from build123d import *

# Parameters (mm, degrees)
F1_DEPTH = 3.175


# Not quite as in the source:
# - a length typed as a fraction of an inch, garbled in the dataset ("3 / 203.2 mm" for 3/8 in), is restored


with BuildPart() as f1:
    # F0 (on Top) → F1 (new body)
    with BuildSketch(Plane.XY):
        with BuildLine():
            ThreePointArc((-41.4974734498, 12.7), (-32.5172173287, 8.9802561211), (-28.7974734498, 0))
            Line((-28.7974734498, 0), (32.2387265502, 0))
            ThreePointArc((32.2387265502, 0), (35.9584704291, 8.9802561211), (44.9387265502, 12.7))
            Line((44.9387265502, 12.7), (-41.4974734498, 12.7))
        make_face()
        with BuildLine():
            ThreePointArc((-41.4974734498, -4.7625), (-44.8650694952, 3.3675960454), (-36.7349734498, 0))
            Line((-36.7349734498, 0), (-28.7974734498, 0))
            ThreePointArc((-28.7974734498, 0), (-32.5172173287, 8.9802561211), (-41.4974734498, 12.7))
            ThreePointArc((-41.4974734498, 12.7), (-54.1974734498, 0), (-41.4974734498, -12.7))
            Line((-41.4974734498, -12.7), (-41.4974734498, -4.7625))
        make_face()
        with BuildLine():
            Line((-28.7974734498, 0), (-36.7349734498, 0))
            ThreePointArc((-36.7349734498, 0), (-38.1298774044, -3.3675960454), (-41.4974734498, -4.7625))
            Line((-41.4974734498, -4.7625), (-41.4974734498, -12.7))
            ThreePointArc((-41.4974734498, -12.7), (-32.5172173287, -8.9802561211), (-28.7974734498, 0))
        make_face()
        with BuildLine():
            Line((32.2387265502, 0), (-28.7974734498, 0))
            ThreePointArc((-28.7974734498, 0), (-32.5172173287, -8.9802561211), (-41.4974734498, -12.7))
            Line((-41.4974734498, -12.7), (44.9387265502, -12.7))
            ThreePointArc((44.9387265502, -12.7), (35.9584704291, -8.9802561211), (32.2387265502, 0))
        make_face()
        with BuildLine():
            ThreePointArc((44.9387265502, 12.7), (35.9584704291, 8.9802561211), (32.2387265502, 0))
            ThreePointArc((32.2387265502, 0), (35.9584704291, -8.9802561211), (44.9387265502, -12.7))
            ThreePointArc((44.9387265502, -12.7), (53.9189826713, -8.9802561211), (57.6387265502, 0))
            ThreePointArc((57.6387265502, 0), (53.9189826713, 8.9802561211), (44.9387265502, 12.7))
        make_face()
        with BuildLine():
            ThreePointArc((49.7012265502, 0), (44.9387265502, -4.7625), (40.1762265502, 0))
            ThreePointArc((40.1762265502, 0), (44.9387265502, 4.7625), (49.7012265502, 0))
        make_face(mode=Mode.SUBTRACT)
    extrude(amount=F1_DEPTH)


solid = f1.part
Geometry check sheet. Reference: the model listing, model coordinates, mm. Give positions to 0.01 mm unless a question says otherwise; leave off trailing zeros. Write each loop counter-clockwise with the first axis right and the second up, starting at its lowest first coordinate (ties: lowest second). Pieces come first, ordered by that corner, then holes. Notation, with made-up numbers: (22.25, 10.25) - (80.25, 10.25) arc R28 cw to (80.25, 32.25) - close; hole circle Ø2 at (81, 89). An arc over 180 degrees is marked (long way). Put each result on its own line as item: value.
1. Draft check along X on faces 1 (the flat face through (1, 0, 0)), 2 (the cylindrical face through (-54.194, 0.279, 1.565)), 3 (the cylindrical face through (-46.255, -0.209, 1.565)). Enter one of: +X half, -X half, draft (parallel to the pull), parting line (faces both ways), or undercut.
Ans:
face 1: draft
face 2: -X half
face 3: undercut
2. Thickness scan on line 1 (X direction, y = 3.75, z = 1.35); line 2 (X direction, y = -0.5, z = 2.5); line 3 (Y direction, x = 48.5, z = 2.05). Record the ranges inside material, lowest first.
Ans:
line 1: x = -53.63 to -44.43, -38.56 to 42, 47.87 to 57.07
line 2: x = -54.19 to -46.23, -36.76 to 40.2, 49.67 to 57.63
line 3: y = -12.19 to -3.16, 3.16 to 12.19
3. Sectioned sample at A-A, the plane z = 1.5. Enter the section's corners in (x, y) (1 decimal).
Ans:
outline: (-41.5, -12.7) - (44.9, -12.7) arc R12.7 ccw to (44.9, 12.7) - (-41.5, 12.7) arc R12.7 ccw to start; hole circle Ø9.5 at (-41.5, 0); hole circle Ø9.5 at (44.9, 0)
4. Sectioned sample at B-B, the plane y = -3.25. Enter the section's corners in (x, z) (1 decimal), plus the area to 3 significant figures.
Ans:
outline: (-53.8, 0) - (-45, 0) - (-45, 3.2) - (-53.8, 3.2) - close; (-38, 0) - (41.5, 0) - (41.5, 3.2) - (-38, 3.2) - close; (48.4, 0) - (57.2, 0) - (57.2, 3.2) - (48.4, 3.2) - close
area: 308 mm²
5. Sectioned sample at D-D, the plane y = 9.75. Enter the section's corners in (x, z) (1 decimal).
Ans:
outline: (-49.6, 0) - (53.1, 0) - (53.1, 3.2) - (-49.6, 3.2) - close
6. Go/stop test with flat-tipped pins: pin 1 (11 mm diameter, centred on x = -41.5, y = 0, fed in from +Z) (3 decimals); pin 2 (7.5 mm diameter, centred on x = 44.94, y = 0, fed in from +Z). Record where each tip stops, or that it passes through.
Ans:
pin 1: stops at z = 3.175
pin 2: passes through
7. Sectioned sample at C-C, the plane y = 1.75. Enter the section's corners in (x, z) (3 decimals).
Ans:
outline: (-54.076, 0) - (-45.927, 0) - (-45.927, 3.175) - (-54.076, 3.175) - close; (-37.068, 0) - (40.509, 0) - (40.509, 3.175) - (-37.068, 3.175) - close; (49.368, 0) - (57.518, 0) - (57.518, 3.175) - (49.368, 3.175) - close
